from build123d import *

# Parameters (mm, degrees)
F0_R     = 35
F1_DEPTH = 4
F2_R     = 28.45
F3_DEPTH = 7
F4_R     = 15.75
F5_DEPTH = 11.001
F6_SIZE  = 1


with BuildPart() as f1:
    # F0 (on Top) → F1 (new body)
    with BuildSketch(Plane.XY):
        Circle(F0_R)
    extrude(amount=F1_DEPTH)

    # F2 (on face) → F3 (join)
    with BuildSketch(Plane.XY.offset(4)):
        Circle(F2_R)
    extrude(amount=F3_DEPTH)

    # F4 (on face) → F5 (cut, through all)
    with BuildSketch(Plane.XY.offset(11)):
        with BuildLine():
            Line((19.520822, 3), (24.265253, 3))
            ThreePointArc((24.265253, 3), (17.288761, 17.288761), (3, 24.265253))
            Line((3, 24.265253), (3, 19.520822))
            ThreePointArc((3, 19.520822), (13.965359, 13.965359), (19.520822, 3))
        make_face()
        with BuildLine():
            ThreePointArc((3, -24.265253), (17.288761, -17.288761), (24.265253, -3))
            Line((24.265253, -3), (19.520822, -3))
            ThreePointArc((19.520822, -3), (13.965359, -13.965359), (3, -19.520822))
            Line((3, -19.520822), (3, -24.265253))
        make_face()
        with BuildLine():
            Line((-3, 19.520822), (-3, 24.265253))
            ThreePointArc((-3, 24.265253), (-17.285086, 17.292435), (-24.263976, 3.010314))
            Line((-24.263976, 3.010314), (-19.514873, 3.038462))
            ThreePointArc((-19.514873, 3.038462), (-13.951592, 13.979112), (-3, 19.520822))
        make_face()
        with BuildLine():
            ThreePointArc((-3.038462, -19.514873), (-13.965359, -13.965359), (-19.514873, -3.038462))
            Line((-19.514873, -3.038462), (-24.263976, -3.010314))
            ThreePointArc((-24.263976, -3.010314), (-17.288467, -17.289054), (-3.00949, -24.264078))
            Line((-3.00949, -24.264078), (-3.038462, -19.514873))
        make_face()
        Circle(F4_R)
    extrude(amount=-F5_DEPTH, mode=Mode.SUBTRACT)

    # F6
    f6_edges = [f1.edges().sort_by_distance(p)[0] for p in [
        (-28.45, 0, 11),
        (-15.75, 0, 0),
    ]]
    chamfer(f6_edges, length=F6_SIZE)


solid = f1.part
Geometry check sheet. Reference: the model listing, model coordinates, mm. A direction names the side the tool comes from. Give positions to 0.01 mm unless a question says otherwise; leave off trailing zeros. Order: outer loops, then holes, each group sorted by start corner. A loop starts at its lowest first (then second) coordinate and runs counter-clockwise, first axis right, second up.
1) Cross-section at C-C (z = 2.5). Record the boundary of the cut face in (x, y).
Results are:
outline: circle Ø70 at (0, 0); hole (-24.26, -3.01) arc R24.45 ccw to (-3.01, -24.26) - (-3.04, -19.51) arc R19.75 cw to (-19.51, -3.04) - close; hole (-24.26, 3.01) - (-19.51, 3.04) arc R19.75 cw to (-3, 19.52) - (-3, 24.27) arc R24.45 ccw to start; hole circle Ø31.5 at (0, 0); hole (3, -24.27) arc R24.45 ccw to (24.27, -3) - (19.52, -3) arc R19.75 cw to (3, -19.52) - close; hole (3, 19.52) arc R19.75 cw to (19.52, 3) - (24.27, 3) arc R24.45 ccw to (3, 24.27) - close
2) Material ranges on probe 1 along Y at (x, z) = (0, 5.5); probe 2 along X at (y, z) = (11.5, 8.75); probe 3 along X at (y, z) = (14, 6.5), recorded low to high.
Results are:
probe 1: y = -28.45 to -15.75, 15.75 to 28.45
probe 2: x = -26.02 to -21.58, -16.06 to -10.76, 10.76 to 16.06, 21.58 to 26.02
probe 3: x = -24.77 to -20.05, -13.93 to -7.22, 7.22 to 13.93, 20.05 to 24.77
3) Draft check along Y on faces 1 (the cylindrical face through (-28, -21, 2)), 2 (the flat face through (0, 29, 4)), 3 (the cylindrical face through (-13.84, -14.09, 5.58)). Enter one of: released by +Y, released by -Y, zero draft, split by the parting line, or undercut.
Results are:
face 1: split by the parting line
face 2: zero draft
face 3: undercut
4) Cross-section at A-A (x = 0). Record the boundary of the cut face in (y, z).
Results are:
outline: (-35, 0) - (-16.75, 0) - (-15.75, 1) - (-15.75, 11) - (-27.45, 11) - (-28.45, 10) - (-28.45, 4) - (-35, 4) - close; (15.75, 1) - (16.75, 0) - (35, 0) - (35, 4) - (28.45, 4) - (28.45, 10) - (27.45, 11) - (15.75, 11) - close
5) Cross-section at D-D (z = 8.75). Record the boundary of the cut face in (x, y), then the cut area to 3 significant figures.
Results are:
outline: circle Ø56.9 at (0, 0); hole (-24.26, -3.01) arc R24.45 ccw to (-3.01, -24.26) - (-3.04, -19.51) arc R19.75 cw to (-19.51, -3.04) - close; hole (-24.26, 3.01) - (-19.51, 3.04) arc R19.75 cw to (-3, 19.52) - (-3, 24.27) arc R24.45 ccw to start; hole circle Ø31.5 at (0, 0); hole (3, -24.27) arc R24.45 ccw to (24.27, -3) - (19.52, -3) arc R19.75 cw to (3, -19.52) - close; hole (3, 19.52) arc R19.75 cw to (19.52, 3) - (24.27, 3) arc R24.45 ccw to (3, 24.27) - close
area: 1,220 mm2
6) Tool access check on faces 4 (the cylindrical face through (27.136, 8.546, 6.958)), 5 (the flat face through (12, -12, 11)), 6 (the flat face through (22, -3, 6)). Record the directions out of +Z, -Z, +X, -X, +Y, -Y that give a thin tool (end or side, any length) a straight path to the whole face; none if there is none.
Results are:
face 4: +Z
face 5: +Z, +X, -X, +Y, -Y
face 6: +Z, -Z
7) Gauge pin test, flat ends, axial feed: pin 1 (5 mm diameter, centred on x = 21.5, z = 5, fed in from +Y); pin 2 (4 mm diameter, centred on x = -10.5, y = 20, fed in from -Z); pin 3 (1 mm diameter, centred on x = -25, z = 9.5, fed in from -Y); pin 4 (4 mm diameter, centred on y = 22, z = 8, fed in from -X). Record the tip position at first contact, or that the pin passes through.
Results are:
pin 1: stops at y = 29.26
pin 2: stops at z = 0
pin 3: stops at y = -14.46
pin 4: stops at x = -20.23
